For this review, use the dimensioned drawing (mm, ordinates from the lowest corner) and the shaded views. Round coordinates to 2 decimals unless told otherwise and drop trailing zeros. Write each loop counter-clockwise with the first axis right and the second up, starting at its lowest first coordinate (ties: lowest second). Pieces come first, ordered by that corner, then holes. Notation, with made-up numbers: M -19.5,29 L 32.5,29 A24 ccw 32.5,53 Z; hole C 60.25,43 d6. An arc over 180 degrees is marked long. Use one line per item in the form item = value. Start each with the question number.
Item 1: For P1, Ø10, axis at x = 56, z = 59, coming from the +Y side, flat-tipped, find the tip position at first contact; note if it passes through.
Item 2: Add section B-B (x = 9.5). State the section outline as (y, z) points.
Item 3: Add section A-A (y = 6.5). State the section outline as (x, z) points, and give its area (3 significant figures).
Item 4: Draft analysis for pull direction X (two halves, no side actions). For the marked faces 1 and 2, state which applies: released by +X, released by -X, zero draft, split by the parting line, or undercut.
Item 5: Add section C-C (z = 46.5). State the section outline as (x, y) points, and give its area (3 significant figures).
Item 6: For line 1 (Z direction, x = 10.5, y = 6); line 2 (X direction, y = 6.75, z = 77.5); line 3 (Y direction, x = 43.5, z = 60), list the stretches that pass through material, from the lowest coordinate up. Write a range as [from, to].
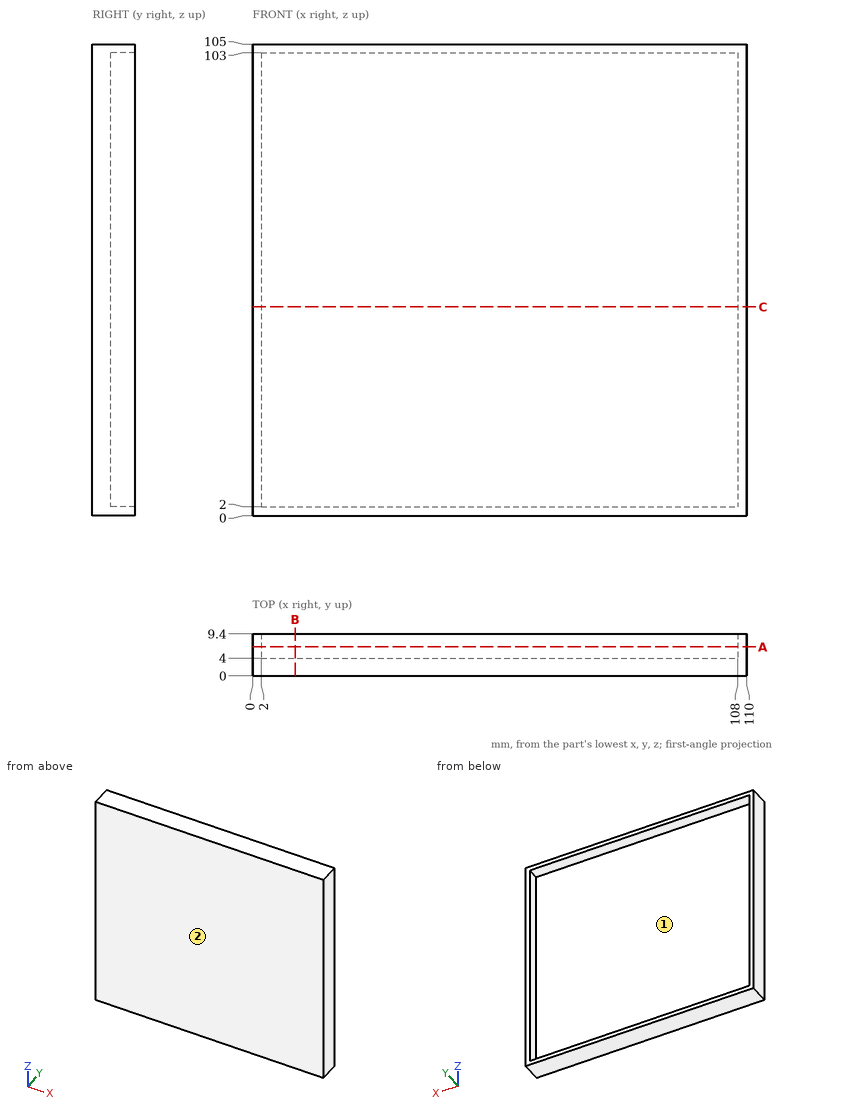
Calculated:
q1.P1 = 4
q2.outline = M 0,0 L 9.4,0 L 9.4,2 L 4,2 L 4,103 L 9.4,103 L 9.4,105 L 0,105 Z
q3.outline = M 0,0 L 110,0 L 110,105 L 0,105 Z; hole M 2,2 L 108,2 L 108,103 L 2,103 Z
q3.area = 844 mm^2
q4.face_1 = undercut
q4.face_2 = zero draft
q5.outline = M 0,0 L 110,0 L 110,9.4 L 108,9.4 L 108,4 L 2,4 L 2,9.4 L 0,9.4 Z
q5.area = 462 mm^2
q6.line_1 = [0, 2], [103, 105]
q6.line_2 = [0, 2], [108, 110]
q6.line_3 = [0, 4]
